Autodesk Inventor part; units mm, degrees
ref_plane "YZ Plane" through (0, 0, 0) normal (1, 0, 0) x (0, 1, 0)
ref_plane "XZ Plane" through (0, 0, 0) normal (0, 1, 0) x (-1, 0, 0)
ref_plane "XY Plane" through (0, 0, 0) normal (0, 0, 1) x (1, 0, 0)
sketch "Sketch1" plane through (0, 0, 0) normal (0, 0, 1) x (1, 0, 0)
  line L0 (0, 0) -> (25.4, 0)
  line L1 (25.4, 0) -> (25.4, 25.4)
  line L2 (25.4, 25.4) -> (22.225, 25.4)
  line L3 (22.225, 25.4) -> (22.225, 3.175)
  line L4 (22.225, 3.175) -> (0, 3.175)
  line L5 (0, 3.175) -> (0, 0)
  dimension "d0" = 3.175
  dimension "d1" = 25.4
extrude "Extrusion1" add sketch "Sketch1" along normal blind 25.4
sketch "Sketch2" plane through (25.4, 0, 0) normal (1, 0, 0) x (0, 0, -1)
  line L0 (0, 0) -> (0, 25.4)
  line L1 (0, 25.4) -> (-25.4, 25.4)
  circle A0 centre (-12.7, 19.05) radius 2.4384
  circle A1 centre (-12.7, 6.35) radius 2.4384
  line L2 (-12.7, 19.05) -> (-12.7, 6.35) construction
  dimension "d4" = 4.8768
  dimension "d5" = 4.8768
  dimension "d6" = 12.7
  dimension "d7" = 12.7
  dimension "d8" = 6.35
extrude "Extrusion2" cut sketch "Sketch2" against normal through all
sketch "Sketch3" plane through (0, 3.175, 0) normal (0, 1, 0) x (1, 0, 0)
  line L0 (0, -25.4) -> (22.225, -25.4)
  line L1 (0, 0) -> (0, -25.4)
  circle A0 centre (12.7, -12.7) radius 7.9375
  dimension "d11" = 12.7
  dimension "d12" = 12.7
  dimension "d13" = 15.875
extrude "Extrusion3" cut sketch "Sketch3" against normal up to next
fillet "Fillet1" radius 3.175 4 edges at (0, 1.5875, 0) (0, 1.5875, 25.4) (23.8125, 25.4, 25.4) (23.8125, 25.4, 0)
sketch "Sketch4" plane through (25.4, 0, 0) normal (0, -1, 0) x (1, 0, 0)
  line L0 (0, 0) -> (0, 25.4)
  arc A0 (0, 25.4) -> (0, 0) centre (139.1215, 12.7) ccw
  line L1 (0, 25.4) -> (0, 0)
  point P0 (-25.4, 0)
  dimension "d17" = 139.7
extrude "Extrusion4" cut sketch "Sketch4" against normal through all
properties part number "HopperMount"
Part model, mm, in its own coordinate system. A direction names the side the tool comes from. Coordinates: 2 decimals unless noted, no trailing zeros. Loops run counter-clockwise (first coordinate to the right, second up) from the corner with the lowest first, then second, coordinate; pieces in that order, holes last. Notation, with made-up numbers: (23.5, 29.25) - (70.5, 29.25) arc R7 ccw to (70.5, 35.25) - close; hole circle Ø11 at (42.25, -33). An arc over 180 degrees is marked (long way). Write each question's results on one line, items separated by ' | '. Start each with the question number.
Q1. Slice it at B-B on x = 12.7. Give the cut face in (y, z) (1 decimal), and give its area (3 significant figures).
Q2. Probe line 1 along Y through (x, z) = (23.35, 12.7); line 2 along Z through (x, y) = (12.7, 2.15); line 3 along Z through (x, y) = (23.35, 19.05). List the from-to ranges inside material, lowest first.
Q3. Two-plate mould, pull along Z, no slides. Class faces 1 (the flat face through (22.5, 7, 0)), 2 (the cylindrical face through (23.79, 24.45, 24.49)), 3 (the cylindrical face through (24.82, 12.52, 12.88)), 4 (the flat face through (0, 2, 13)): +Z half, -Z half, draft (parallel to the pull), parting line (faces both ways), or undercut.
Q4. Which spindle directions (+Z, -Z, +X, -X, +Y, -Y) get a long thin tool onto all of the face, cutting with end or side? Do faces 5 (the flat face through (4, 3.175, 13)), 6 (the cylindrical face through (11.67, 1.61, 4.83)). Say none if no direction does.
Q5. Slice it at C-C on z = 12.7. Give the cut face in (x, y) (1 decimal).
Q6. Drop flat-ended pins along their axis: pin 1 Ø6 at (y, z) = (14.5, 18) entering from -X (3 decimals); pin 2 Ø4 at (y, z) = (6.35, 12.7) entering from +X; pin 3 Ø5 at (x, z) = (3, 14) entering from +Y (3 decimals); pin 4 Ø2 at (y, z) = (11, 14.5) entering from +X. Give the stop position or say it passes through.
Q7. Slice it at A-A on y = 6.35. Give the cut face in (x, z) (1 decimal).
Answer:
1) outline: (0, 0) - (3.2, 0) - (3.2, 4.8) - (0, 4.8) - close; (0, 20.6) - (3.2, 20.6) - (3.2, 25.4) - (0, 25.4) - close | area: 30.2 mm2
2) line 1: y = 0 to 3.91, 8.79 to 16.61, 21.49 to 25.4 | line 2: z = 0 to 4.76, 20.64 to 25.4 | line 3: z = 0 to 10.26, 15.14 to 25.4
3) face 1: -Z half | face 2: +Z half | face 3: undercut | face 4: draft
4) face 5: +Z, -Z, -X, +Y | face 6: +Y, -Y
5) outline: (0, 0) - (4.8, 0) - (4.8, 3.2) - (0, 3.2) - close; (20.6, 0) - (24.8, 0) - (24.8, 3.9) - (22.2, 3.9) - (22.2, 3.2) - (20.6, 3.2) - close; (22.2, 8.8) - (24.8, 8.8) - (24.8, 16.6) - (22.2, 16.6) - close; (22.2, 21.5) - (24.8, 21.5) - (24.8, 25.4) - (22.2, 25.4) - close
6) pin 1: stops at x = 22.225 | pin 2: passes through | pin 3: stops at y = 3.175 | pin 4: stops at x = 24.85
7) outline: (22.2, 0) - (25.4, 0) arc R139.7 cw to (24.8, 10.3) - (22.2, 10.3) - close; (22.2, 15.1) - (24.8, 15.1) arc R139.7 cw to (25.4, 25.4) - (22.2, 25.4) - close
